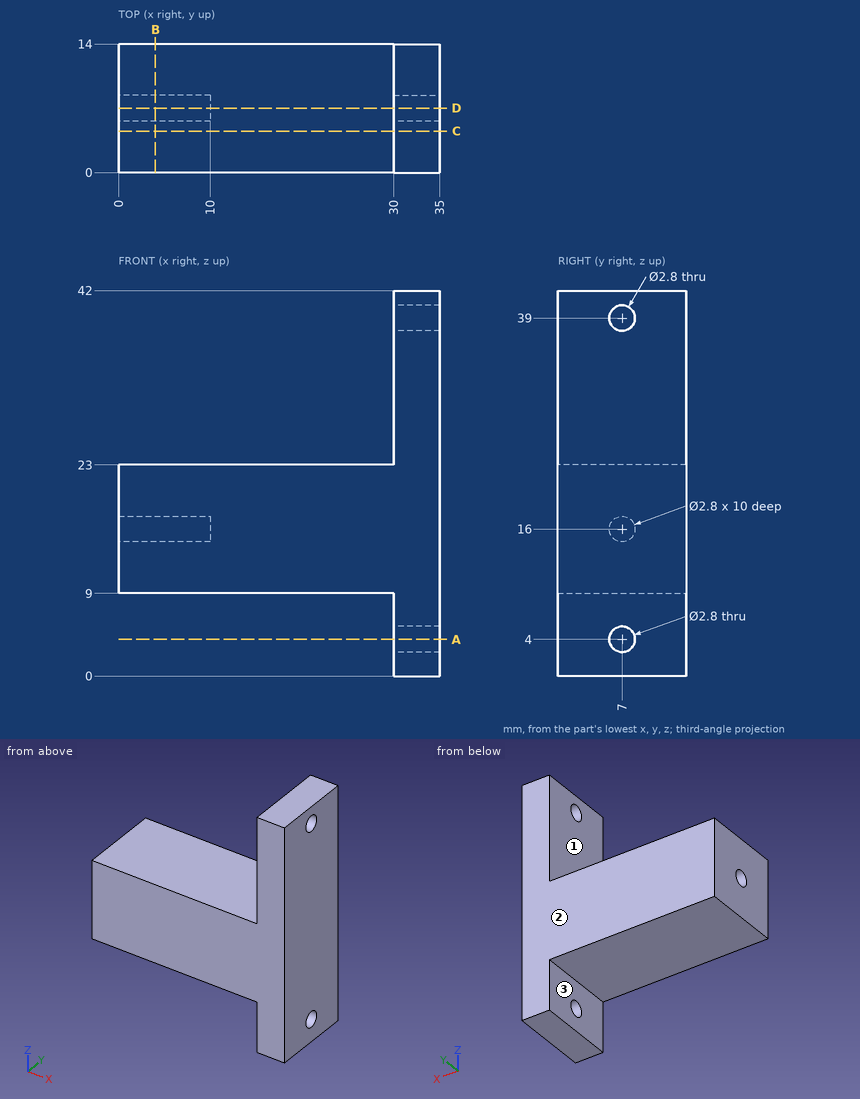
Check sheet for the drawn part. Datum: minimum x, y, z corner. Units: mm. A direction names the side the tool comes from. Coordinates: 2 decimals unless noted, no trailing zeros. Loops run counter-clockwise (first coordinate to the right, second up) from the corner with the lowest first, then second, coordinate; pieces in that order, holes last. Notation, with made-up numbers: (83, 44) -> (92, 44) arc R6 ccw to (92, 53) -> close; hole circle Ø8 at (79.25, 83). An arc over 180 degrees is marked (long way). Answer as a JSON object with one key per item and string values. Group by question number.
Item 1: Depth check by flat-ended pin: pin 1 (1 mm diameter, centred on y = 9.5, z = 7.5, fed in from -X); pin 2 (0.8 mm diameter, centred on y = 7.5, z = 16.5, fed in from -X); pin 3 (2 mm diameter, centred on x = 16.5, y = 11, fed in from -Z); pin 4 (2.5 mm diameter, centred on y = 7, z = 39, fed in from +X). Enter the tip coordinate at first touch or a pass-through.
Item 2: Tool access check on the marked faces 1, 2 and 3. Record the directions out of +Z, -Z, +X, -X, +Y, -Y that give a thin tool (end or side, any length) a straight path to the whole face; none if there is none.
Item 3: Scan lines: probe 1 along Z at (x, y) = (32.6, 7); probe 2 along Y at (x, z) = (6, 16); probe 3 along Z at (x, y) = (21.5, 2.25). Record each from-to range of solid material in increasing order.
Item 4: Sectioned sample at A-A on z = 4. Record the boundary of the cut face in (x, y), plus the area to 3 significant figures.
Item 5: Sectioned sample at C-C on y = 4.5. Record the boundary of the cut face in (x, z), plus the area to 3 significant figures.
Item 6: Sectioned sample at D-D on y = 7. Record the boundary of the cut face in (x, z).
Item 7: Sectioned sample at B-B on x = 4. Record the boundary of the cut face in (y, z).
Evaluation:
{
 "1": {"pin 1": "stops at x = 30", "pin 2": "stops at x = 10", "pin 3": "stops at z = 9", "pin 4": "passes through"},
 "2": {"face 1": "+Z, -X, +Y, -Y", "face 2": "+Z, -Z, +X, -X, +Y", "face 3": "-Z, -X, +Y, -Y"},
 "3": {"probe 1": "z = 0 to 2.6, 5.4 to 37.6, 40.4 to 42", "probe 2": "y = 0 to 5.6, 8.4 to 14", "probe 3": "z = 9 to 23"},
 "4": {"outline": "(30, 0) -> (35, 0) -> (35, 5.6) -> (30, 5.6) -> close; (30, 8.4) -> (35, 8.4) -> (35, 14) -> (30, 14) -> close", "area": "56.0 mm²"},
 "5": {"outline": "(0, 9) -> (30, 9) -> (30, 0) -> (35, 0) -> (35, 42) -> (30, 42) -> (30, 23) -> (0, 23) -> close", "area": "630 mm²"},
 "6": {"outline": "(0, 9) -> (30, 9) -> (30, 5.4) -> (35, 5.4) -> (35, 37.6) -> (30, 37.6) -> (30, 23) -> (0, 23) -> (0, 17.4) -> (10, 17.4) -> (10, 14.6) -> (0, 14.6) -> close; (30, 0) -> (35, 0) -> (35, 2.6) -> (30, 2.6) -> close; (30, 40.4) -> (35, 40.4) -> (35, 42) -> (30, 42) -> close"},
 "7": {"outline": "(0, 9) -> (14, 9) -> (14, 23) -> (0, 23) -> close; hole circle Ø2.8 at (7, 16)"}
}
